```python
from build123d import *

# Parameters (mm, degrees)
SKETCH1_W           = 27.95
SKETCH1_H           = 13.5
BOSS_EXTRUDE1_DEPTH = 1.5
SKETCH2_W           = 21.7
SKETCH2_H           = 10.8
CUT_EXTRUDE1_DEPTH  = 0.2
SKETCH3_W           = 23.7
SKETCH3_H           = 12.8
CUT_EXTRUDE2_DEPTH  = 0.1


with BuildPart() as part:
    # Sketch1 → Boss-Extrude1 (new body)
    with BuildSketch(Plane(origin=(0, 0, 0), x_dir=(1, 0, 0), z_dir=(0, 1, 0))):
        with Locations((-1.425, 0)):
            Rectangle(SKETCH1_W, SKETCH1_H)
    extrude(amount=BOSS_EXTRUDE1_DEPTH)

    # Sketch2 → Cut-Extrude1 (cut)
    with BuildSketch(Plane(origin=(0, 1.5, 0), x_dir=(1, 0, 0), z_dir=(0, 1, 0))):
        Rectangle(SKETCH2_W, SKETCH2_H)
    extrude(amount=-CUT_EXTRUDE1_DEPTH, mode=Mode.SUBTRACT)

    # Sketch3 → Cut-Extrude2 (cut)
    with BuildSketch(Plane(origin=(0, 1.5, 0), x_dir=(1, 0, 0), z_dir=(0, 1, 0))):
        Rectangle(SKETCH3_W, SKETCH3_H)
    extrude(amount=-CUT_EXTRUDE2_DEPTH, mode=Mode.SUBTRACT)


solid = part.part
```
The model under review builds one solid part; all positions refer to its coordinate system, in mm. Coordinates: 2 decimals unless noted, no trailing zeros. Write each loop counter-clockwise with the first axis right and the second up, starting at its lowest first coordinate (ties: lowest second). Pieces come first, ordered by that corner, then holes. Notation, with made-up numbers: (-29.75, 10) - (-16.75, 10) arc R18 ccw to (-16.75, 39) - close; hole circle Ø2 at (-11, 63.5). An arc over 180 degrees is marked (long way). Answer in a Markdown table with one row per item. Add a question column.
Q1. Consider section A-A on x = -9. Give the boundary of the cut face in (y, z).
Q2. To check wall thickness, follow line 1 along Y through (x, z) = (-6.5, 2.5); line 2 along Y through (x, z) = (4.5, 5.5). State the ranges of each line that lie inside material, in increasing order. Write a range as from..to.
Q3. Clearance check with a flat-ended pin moving along its axis: pin 1 (1 mm diameter, centred on x = 2.5, z = -3.5, fed in from +Y). State where the tip first meets the part, or that it passes through.
Q4. Consider section C-C on z = 5.75. Give the boundary of the cut face in (x, y).
Q5. Draft analysis for pull direction X (two halves, no side actions). For faces 1 (the face through (12.55, 1, 0)), 2 (the face through (-2, 1, 6.75)), 3 (the face through (-1, 1.4, 6)), 4 (the face through (0, 1.3, 0)), state which applies: +X half, -X half, draft (parallel to the pull), parting line (faces both ways), or undercut.
Q6. Consider section B-B on z = 0.5. Give the boundary of the cut face in (x, y).
Answers below:
| question | item | result |
|---|---|---|
| 1 | outline | (0, -6.75) - (1.5, -6.75) - (1.5, -6.4) - (1.4, -6.4) - (1.4, -5.4) - (1.3, -5.4) - (1.3, 5.4) - (1.4, 5.4) - (1.4, 6.4) - (1.5, 6.4) - (1.5, 6.75) - (0, 6.75) - close |
| 2 | line 1 | 0..1.3 |
| 2 | line 2 | 0..1.4 |
| 3 | pin 1 | y = 1.3 |
| 4 | outline | (-15.4, 0) - (12.55, 0) - (12.55, 1.5) - (11.85, 1.5) - (11.85, 1.4) - (-11.85, 1.4) - (-11.85, 1.5) - (-15.4, 1.5) - close |
| 5 | face 1 | +X half |
| 5 | face 2 | draft |
| 5 | face 3 | undercut |
| 5 | face 4 | undercut |
| 6 | outline | (-15.4, 0) - (12.55, 0) - (12.55, 1.5) - (11.85, 1.5) - (11.85, 1.4) - (10.85, 1.4) - (10.85, 1.3) - (-10.85, 1.3) - (-10.85, 1.4) - (-11.85, 1.4) - (-11.85, 1.5) - (-15.4, 1.5) - close |
